Check sheet for the modelled part. Datum: model origin and axes. Units: mm. Round coordinates to 2 decimals unless told otherwise and drop trailing zeros. One line per item, written item: value.
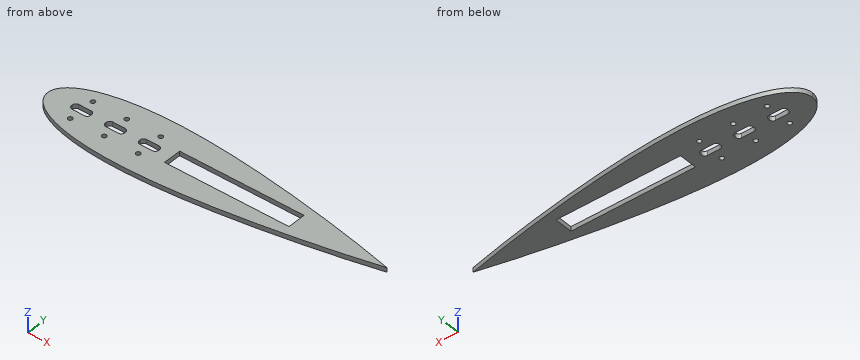
from build123d import *

# Parameters (mm, degrees)
SKETCH_1_R      = 2
SKETCH_1_W      = 110
SKETCH_1_H      = 16
EXTRUDE_1_DEPTH = 4


with BuildPart() as part:
    # 草图1 → 凸台-拉伸1 (new body)
    with BuildSketch(Plane.XY):
        with BuildLine():
            add(Edge.make_bspline(
                [(0, 0), (-0.00021229, 0.506970744), (0.044864754, 1.381714413), (0.226017079, 2.650839475), (0.688025344, 4.299952552), (1.335546305, 5.873041675), (2.26695445, 7.542579189), (3.571946964, 9.346109572), (5.391381815, 11.324673938), (7.954469743, 13.539518757), (11.584975672, 16.021510412), (16.648123966, 18.726988569), (23.793189999, 21.649781435), (33.085765079, 24.436937203), (46.643058908, 27.284493785), (64.063199307, 29.362693495), (84.450847037, 30.260343335), (107.414943041, 29.859960777), (130.332556147, 28.428346139), (153.186136376, 26.214758658), (175.970846287, 23.391654718), (195.848592789, 20.487628812), (212.844945694, 17.732999103), (226.980485609, 15.27094618), (238.271313866, 13.203878393), (248.135151077, 11.310105462), (256.577305747, 9.625486685), (263.604664912, 8.179483676), (269.219788458, 6.997398786), (274.1309907, 5.93944771), (278.331979904, 5.017052178), (281.838528118, 4.234963306), (284.626645762, 3.606112196), (287.446648095, 2.96209323), (290.200347561, 2.326575377), (293.076089097, 1.653806717), (295.700233888, 1.034172197), (298.078453529, 0.464134201), (299.36547076, 0.153714708), (299.999999999, 0)],
                knots=[0, 0, 0, 0, 0, 0.005874531, 0.010168378, 0.014828146, 0.019835444, 0.025574736, 0.032308878, 0.040609511, 0.050966894, 0.064812119, 0.083253248, 0.107120705, 0.140429682, 0.177263566, 0.243881637, 0.310499708, 0.377117784, 0.443735861, 0.510353937, 0.576972013, 0.643590091, 0.67689913, 0.710208169, 0.743517207, 0.776826246, 0.793480766, 0.810135286, 0.826789806, 0.843444325, 0.851771585, 0.860098845, 0.868426105, 0.876753365, 0.885080625, 0.893407884, 0.901735144, 0.910062404, 0.910062404, 0.910062404, 0.910062404, 0.910062404], degree=4))
            add(Edge.make_bspline(
                [(0, 0), (-0.00021229, -0.506970744), (0.044864754, -1.381714413), (0.226017079, -2.650839475), (0.688025344, -4.299952552), (1.335546305, -5.873041675), (2.26695445, -7.542579189), (3.571946964, -9.346109572), (5.391381815, -11.324673938), (7.954469743, -13.539518757), (11.584975672, -16.021510412), (16.648123966, -18.726988569), (23.793189999, -21.649781435), (33.085765079, -24.436937203), (46.643058908, -27.284493785), (64.063199307, -29.362693495), (84.450847037, -30.260343335), (107.414943041, -29.859960777), (130.332556147, -28.428346139), (153.186136376, -26.214758658), (175.970846287, -23.391654718), (195.848592789, -20.487628812), (212.844945694, -17.732999103), (226.980485609, -15.27094618), (238.271313866, -13.203878393), (248.135151077, -11.310105462), (256.577305747, -9.625486685), (263.604664912, -8.179483676), (269.219788458, -6.997398786), (274.1309907, -5.93944771), (278.331979904, -5.017052178), (281.838528118, -4.234963306), (284.626645762, -3.606112196), (287.446648095, -2.96209323), (290.200347561, -2.326575377), (293.076089097, -1.653806717), (295.700233888, -1.034172197), (298.078453528, -0.464134202), (299.36547076, -0.153714708), (299.999999999, 0)],
                knots=[0, 0, 0, 0, 0, 0.005874531, 0.010168378, 0.014828146, 0.019835444, 0.025574736, 0.032308878, 0.040609511, 0.050966894, 0.064812119, 0.083253248, 0.107120705, 0.140429682, 0.177263566, 0.243881637, 0.310499708, 0.377117784, 0.443735861, 0.510353937, 0.576972013, 0.643590091, 0.67689913, 0.710208169, 0.743517207, 0.776826246, 0.793480766, 0.810135286, 0.826789806, 0.843444325, 0.851771585, 0.860098845, 0.868426105, 0.876753365, 0.885080625, 0.893407884, 0.901735144, 0.910062404, 0.910062404, 0.910062404, 0.910062404, 0.910062404], degree=4))
        make_face()
        with Locations((30, 12)):
            Circle(SKETCH_1_R, mode=Mode.SUBTRACT)
        with Locations((30, -12)):
            Circle(SKETCH_1_R, mode=Mode.SUBTRACT)
        with Locations((60, 12)):
            Circle(SKETCH_1_R, mode=Mode.SUBTRACT)
        with Locations((60, -12)):
            Circle(SKETCH_1_R, mode=Mode.SUBTRACT)
        with Locations((90, 12)):
            Circle(SKETCH_1_R, mode=Mode.SUBTRACT)
        with Locations((90, -12)):
            Circle(SKETCH_1_R, mode=Mode.SUBTRACT)
        with BuildLine():
            Line((54.5, 3.5), (65.5, 3.5))
            ThreePointArc((65.5, 3.5), (67.621320344, 2.621320344), (68.5, 0.5))
            Line((68.5, 0.5), (68.5, -0.5))
            ThreePointArc((68.5, -0.5), (67.621320344, -2.621320344), (65.5, -3.5))
            Line((65.5, -3.5), (54.5, -3.5))
            ThreePointArc((54.5, -3.5), (52.378679656, -2.621320344), (51.5, -0.5))
            Line((51.5, -0.5), (51.5, 0.5))
            ThreePointArc((51.5, 0.5), (52.378679656, 2.621320344), (54.5, 3.5))
        make_face(mode=Mode.SUBTRACT)
        with BuildLine():
            Line((24.5, 3.5), (35.5, 3.5))
            ThreePointArc((35.5, 3.5), (37.621320344, 2.621320344), (38.5, 0.5))
            Line((38.5, 0.5), (38.5, -0.5))
            ThreePointArc((38.5, -0.5), (37.621320344, -2.621320344), (35.5, -3.5))
            Line((35.5, -3.5), (24.5, -3.5))
            ThreePointArc((24.5, -3.5), (22.378679656, -2.621320344), (21.5, -0.5))
            Line((21.5, -0.5), (21.5, 0.5))
            ThreePointArc((21.5, 0.5), (22.378679656, 2.621320344), (24.5, 3.5))
        make_face(mode=Mode.SUBTRACT)
        with BuildLine():
            Line((84.5, 3.5), (95.5, 3.5))
            ThreePointArc((95.5, 3.5), (97.621320344, 2.621320344), (98.5, 0.5))
            Line((98.5, 0.5), (98.5, -0.5))
            ThreePointArc((98.5, -0.5), (97.621320344, -2.621320344), (95.5, -3.5))
            Line((95.5, -3.5), (84.5, -3.5))
            ThreePointArc((84.5, -3.5), (82.378679656, -2.621320344), (81.5, -0.5))
            Line((81.5, -0.5), (81.5, 0.5))
            ThreePointArc((81.5, 0.5), (82.378679656, 2.621320344), (84.5, 3.5))
        make_face(mode=Mode.SUBTRACT)
        with Locations((165, 0)):
            Rectangle(SKETCH_1_W, SKETCH_1_H, mode=Mode.SUBTRACT)
    extrude(amount=EXTRUDE_1_DEPTH)


solid = part.part
Item 1: Material ranges on line 1 along Y through (x, z) = (60, 2.7); line 2 along Y through (x, z) = (86.5, 0.5); line 3 along Y through (x, z) = (228, 3.3), recorded low to high.
Result set:
line 1: -28.69 to -14, -10 to -3.5, 3.5 to 10, 14 to 28.69
line 2: -29.99 to -3.5, 3.5 to 29.99
line 3: -15.07 to 15.07
Item 2: Sectioned sample at A-A (z = 2.3). State how many separate pieces and enclosed holes the cut face has, then the cut area to 3 significant figures.
Result set:
separate pieces: 1
enclosed holes: 10
area: 10,100 mm^2
Item 3: Depth check by flat-ended pin: pin 1 (2 mm diameter, centred on x = 60.5, z = 1, fed in from +Y); pin 2 (2 mm diameter, centred on x = 157, z = 2.5, fed in from +Y); pin 3 (1.2 mm diameter, centred on x = 145, z = 1, fed in from -Y). Enter the tip coordinate at first touch or a pass-through.
Result set:
pin 1: y = 28.83
pin 2: y = 25.77
pin 3: y = -27.01
